Could you check a few things on this model? Use its own coordinates, in mm. A direction names the side the tool comes from. Coordinates: 2 decimals unless noted, no trailing zeros. Order: outer loops, then holes, each group sorted by start corner. A loop starts at its lowest first (then second) coordinate and runs counter-clockwise, first axis right, second up. Notation, with made-up numbers: (78.5, 45) -> (85.5, 45) arc R15 cw to (85.5, 53) -> close; hole circle Ø5 at (-36, -40). An arc over 180 degrees is marked (long way). Put each result on its own line as item: value. Start each with the question number.
Q1. We'd pull the mould along Y, two halves only. Please class faces 1 (the face through (23.5, 8.07, 5.07)), 2 (the face through (0, 22, 5)), 3 (the face through (24.7, 45, 7.2)): +Y half, -Y half, draft (parallel to the pull), parting line (faces both ways), or undercut.
Q2. If we section it at A-A (y = 22.5): Please give me the cut outline in (x, z), and give its area (3 significant figures).
Q3. Please list where these lines run through material, in increasing order: line 1 along X through (y, z) = (42.5, 1.5); line 2 along X through (y, z) = (22, 9.25); line 3 along Y through (x, z) = (25, 2).
Q4. If we section it at D-D (z = 3.25): Please give me the cut outline in (x, y) (3 decimals).
Q5. If we section it at B-B (x = 25): Please give me the cut outline in (y, z), and give its area (4 significant figures).
Q6. If we section it at C-C (y = 39): Please give me the cut outline in (x, z).
Q7. For faces 4 (the face through (30.537, 11.854, 5.07)), 5 (the face through (25, 39, 7)), which set-ups out of +Z, -Z, +X, -X, +Y, -Y let a thin tool reach every point of the face, with its end or its side?
from build123d import *

# Parameters (mm, degrees)
ESQUISSE1_W      = 50
ESQUISSE1_H      = 10
EXTRUSION1_DEPTH = 45
ESQUISSE2_R      = 12
ESQUISSE2_R_2    = 1.5
EXTRUSION2_DEPTH = 45
EXTRUSION5_DEPTH = 7


with BuildPart() as part:
    # Esquisse1 → Extrusion1 (new body)
    with BuildSketch(Plane(origin=(0, 0, 0), x_dir=(1, 0, 0), z_dir=(0, 1, 0))):
        with Locations((25, -5)):
            Rectangle(ESQUISSE1_W, ESQUISSE1_H)
    extrude(amount=EXTRUSION1_DEPTH)

    # Esquisse2 → Extrusion2 (cut)
    with BuildSketch(Plane.XY.offset(10)):
        with Locations((25, 22.5)):
            Circle(ESQUISSE2_R)
        with Locations((12.445, 29.74863263)):
            Circle(ESQUISSE2_R_2)
        with Locations((37.555, 29.74863263)):
            Circle(ESQUISSE2_R_2)
        with Locations((25, 8.002734741)):
            Circle(ESQUISSE2_R_2)
    extrude(amount=-EXTRUSION2_DEPTH, mode=Mode.SUBTRACT)

    # Esquisse3 → Extrusion5 (cut)
    with BuildSketch(Plane.XY):
        with BuildLine():
            Line((30, 33.408712115), (30, 45))
            Line((30, 45), (20, 45))
            Line((20, 45), (20, 33.408712115))
            ThreePointArc((20, 33.408712115), (25, 34.5), (30, 33.408712115))
        make_face()
    extrude(amount=EXTRUSION5_DEPTH, mode=Mode.SUBTRACT)


solid = part.part
The answers:
1. face 1: undercut
1. face 2: draft
1. face 3: +Y half
2. outline: (0, 0) -> (13, 0) -> (13, 10) -> (0, 10) -> close; (37, 0) -> (50, 0) -> (50, 10) -> (37, 10) -> close
2. area: 260 mm^2
3. line 1: 0 to 20, 30 to 50
3. line 2: 0 to 13.01, 36.99 to 50
3. line 3: 0 to 6.5, 9.5 to 10.5
4. outline: (0, 0) -> (50, 0) -> (50, 45) -> (30, 45) -> (30, 33.409) arc R12 cw (long way) to (20, 33.409) -> (20, 45) -> (0, 45) -> close; hole circle Ø3 at (12.445, 29.749); hole circle Ø3 at (25, 8.003); hole circle Ø3 at (37.555, 29.749)
5. outline: (0, 0) -> (6.5, 0) -> (6.5, 10) -> (0, 10) -> close; (9.5, 0) -> (10.5, 0) -> (10.5, 10) -> (9.5, 10) -> close; (34.5, 7) -> (45, 7) -> (45, 10) -> (34.5, 10) -> close
5. area: 106.5 mm^2
6. outline: (0, 0) -> (20, 0) -> (20, 7) -> (30, 7) -> (30, 0) -> (50, 0) -> (50, 10) -> (0, 10) -> close
7. face 4: +Z, -Z
7. face 5: -Z, +Y
